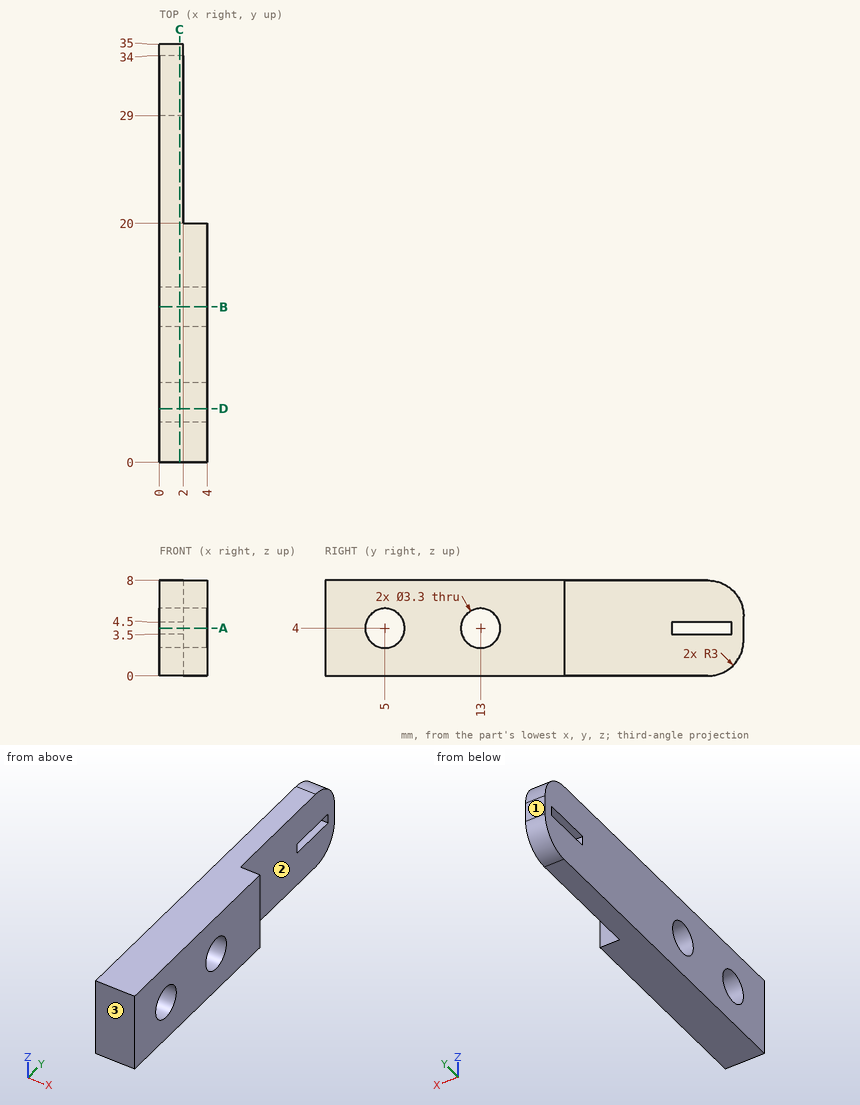
Could you check a few things on this drawing? It's one solid part, dimensions in mm from its lowest x, y, z. Round coordinates to 2 decimals unless told otherwise and drop trailing zeros. Loops run counter-clockwise (first coordinate to the right, second up) from the corner with the lowest first, then second, coordinate; pieces in that order, holes last.
Q1. I want a section at C-C (x = 1.7). Write out the boundary of the cut face in (y, z).
Q2. I want a section at B-B (y = 13). Write out the boundary of the cut face in (x, z), and give its area (3 significant figures).
Q3. Thinking about a two-plate mould opening in Y: for the marked faces 1, 2 and 3, which applies, pulls with the +Y half, pulls with the -Y half, needs draft (parallel to the pull), parting line crosses it, or undercut?
Q4. Please list where these lines run through material, in increasing order: L1, parallel to Y at x = 1.55, z = 5; L2, parallel to Z at x = 2.6, y = 13; L3, parallel to Y at x = 2.55, z = 4.5.
Q5. I want a section at D-D (y = 4.5). Write out the boundary of the cut face in (x, z).
Q6. For P1, Ø2, axis at x = 2.5, z = 3.5, coming from the +Y side; P2, Ø2.5, axis at y = 5, z = 4, coming from the +X side; P3, Ø4, axis at y = 28, z = 5.5, coming from the +X side, each with a flat end and sliding along its axis, tell me the tip position at first contact or that it passes through.
Q7. I want a section at A-A (z = 4). Write out the boundary of the cut face in (x, y), and give its area (3 significant figures).
Answer below:
1. outline: (0, 0) - (32, 0) arc R3 ccw to (35, 3) - (35, 5) arc R3 ccw to (32, 8) - (0, 8) - close; hole circle Ø3.3 at (5, 4); hole circle Ø3.3 at (13, 4); hole (29, 3.5) - (34, 3.5) - (34, 4.5) - (29, 4.5) - close
2. outline: (0, 0) - (4, 0) - (4, 2.35) - (0, 2.35) - close; (0, 5.65) - (4, 5.65) - (4, 8) - (0, 8) - close
2. area: 18.8 mm2
3. face 1: pulls with the +Y half
3. face 2: needs draft
3. face 3: pulls with the -Y half
4. L1: y = 0 to 3.69, 6.31 to 11.69, 14.31 to 35
4. L2: z = 0 to 2.35, 5.65 to 8
4. L3: y = 0 to 3.43, 6.57 to 11.43, 14.57 to 20
5. outline: (0, 0) - (4, 0) - (4, 2.43) - (0, 2.43) - close; (0, 5.57) - (4, 5.57) - (4, 8) - (0, 8) - close
6. P1: stops at y = 35
6. P2: passes through
6. P3: stops at x = 2
7. outline: (0, 0) - (4, 0) - (4, 3.35) - (0, 3.35) - close; (0, 6.65) - (4, 6.65) - (4, 11.35) - (0, 11.35) - close; (0, 14.65) - (4, 14.65) - (4, 20) - (2, 20) - (2, 29) - (0, 29) - close; (0, 34) - (2, 34) - (2, 35) - (0, 35) - close
7. area: 73.6 mm2
